Read the model definition and answer for the solid it produces. Units are mm, in the model's axes. Coordinates: 2 decimals unless noted, no trailing zeros. Write each loop counter-clockwise with the first axis right and the second up, starting at its lowest first coordinate (ties: lowest second). Pieces come first, ordered by that corner, then holes.
(1) The mould has two halves that part along Z. Classify faces 1 (the cylindrical face through (-294.297, 1.521, -6.014)), 2 (the flat face through (-152, 0, -61)), 3 (the cylindrical face through (-6.014, 1.521, -114.297)), 4 (the cylindrical face through (-244.846, 1.479, -37.999)): +Z half, -Z half, draft (parallel to the pull), parting line (faces both ways), or undercut.
(2) Find the intervals of material crossed by probe 1 along Z at (x, y) = (-252, 2); probe 2 along Z at (x, y) = (-283, 1.15); probe 3 along X at (y, z) = (1.4, -108), in increasing order.
(3) Section A-A on x = -252 is taken. Write down the section's boundary in (y, z).
(4) Section B-B on y = 1.45 is taken. State how many separate pieces and enclosed holes the cut face has, then the cut area to 3 significant figures.
from build123d import *

# Parameters (mm, degrees)
SKETCH_2_W      = 300
SKETCH_2_H      = 120
SKETCH_2_R      = 1.5
SKETCH_2_R_2    = 2
SKETCH_2_R_3    = 7.5
SKETCH_2_W_2    = 13
SKETCH_2_H_2    = 6
EXTRUDE_1_DEPTH = 3
FILLET_1_R      = 20


with BuildPart() as part:
    # Эскиз2 → Бобышка-Вытянуть1 (new body)
    with BuildSketch(Plane(origin=(0, 0, 0), x_dir=(1, 0, 0), z_dir=(0, 1, 0))):
        with Locations((-150, 60)):
            Rectangle(SKETCH_2_W, SKETCH_2_H)
        with Locations((-283, 108)):
            Circle(SKETCH_2_R, mode=Mode.SUBTRACT)
        with Locations((-17, 108)):
            Circle(SKETCH_2_R_2, mode=Mode.SUBTRACT)
        with Locations((-17, 12)):
            Circle(SKETCH_2_R, mode=Mode.SUBTRACT)
        with Locations((-283, 12)):
            Circle(SKETCH_2_R, mode=Mode.SUBTRACT)
        with Locations((-252, 35.746485704)):
            Circle(SKETCH_2_R_3, mode=Mode.SUBTRACT)
        with Locations((-207, 43.496485704)):
            Rectangle(SKETCH_2_W_2, SKETCH_2_H_2, mode=Mode.SUBTRACT)
        with BuildLine():
            Line((-173.9, 39.324194468), (-173.9, 32.16877694))
            ThreePointArc((-173.9, 32.16877694), (-172.022697555, 30.140426091), (-169.5, 29.011502408))
            Line((-169.5, 29.011502408), (-169.5, 34.496485704))
            Line((-169.5, 34.496485704), (-166.5, 34.496485704))
            Line((-166.5, 34.496485704), (-166.5, 29.011502408))
            ThreePointArc((-166.5, 29.011502408), (-163.977302445, 30.140426091), (-162.1, 32.16877694))
            Line((-162.1, 32.16877694), (-162.1, 39.324194468))
            ThreePointArc((-162.1, 39.324194468), (-163.977302445, 41.352545317), (-166.5, 42.481469))
            Line((-166.5, 42.481469), (-166.5, 36.996485704))
            Line((-166.5, 36.996485704), (-169.5, 36.996485704))
            Line((-169.5, 36.996485704), (-169.5, 42.481469))
            ThreePointArc((-169.5, 42.481469), (-172.022697555, 41.352545317), (-173.9, 39.324194468))
        make_face(mode=Mode.SUBTRACT)
    extrude(amount=EXTRUDE_1_DEPTH)

    # Скругление1
    fillet_1_edges = [part.edges().sort_by_distance(p)[0] for p in [
        (0, 1.5, 0),
        (-300, 1.5, 0),
        (-300, 1.5, -120),
        (0, 1.5, -120),
    ]]
    fillet(fillet_1_edges, radius=FILLET_1_R)


solid = part.part
Response:
1. face 1: +Z half
1. face 2: draft
1. face 3: -Z half
1. face 4: undercut
2. probe 1: z = -120 to -43.25, -28.25 to 0
2. probe 2: z = -119.77 to -109.5, -106.5 to -13.5, -10.5 to -0.23
2. probe 3: x = -298.33 to -284.5, -281.5 to -19, -15 to -1.67
3. outline: (0, -120) - (3, -120) - (3, -43.25) - (0, -43.25) - close; (0, -28.25) - (3, -28.25) - (3, 0) - (0, 0) - close
4. separate pieces: 1
4. enclosed holes: 7
4. area: 35,300 mm2
